Part print with two shaded views. Sizes in mm from the minimum x, y, z corner. Coordinates: 2 decimals unless noted, no trailing zeros. Order: outer loops, then holes, each group sorted by start corner. A loop starts at its lowest first (then second) coordinate and runs counter-clockwise, first axis right, second up.
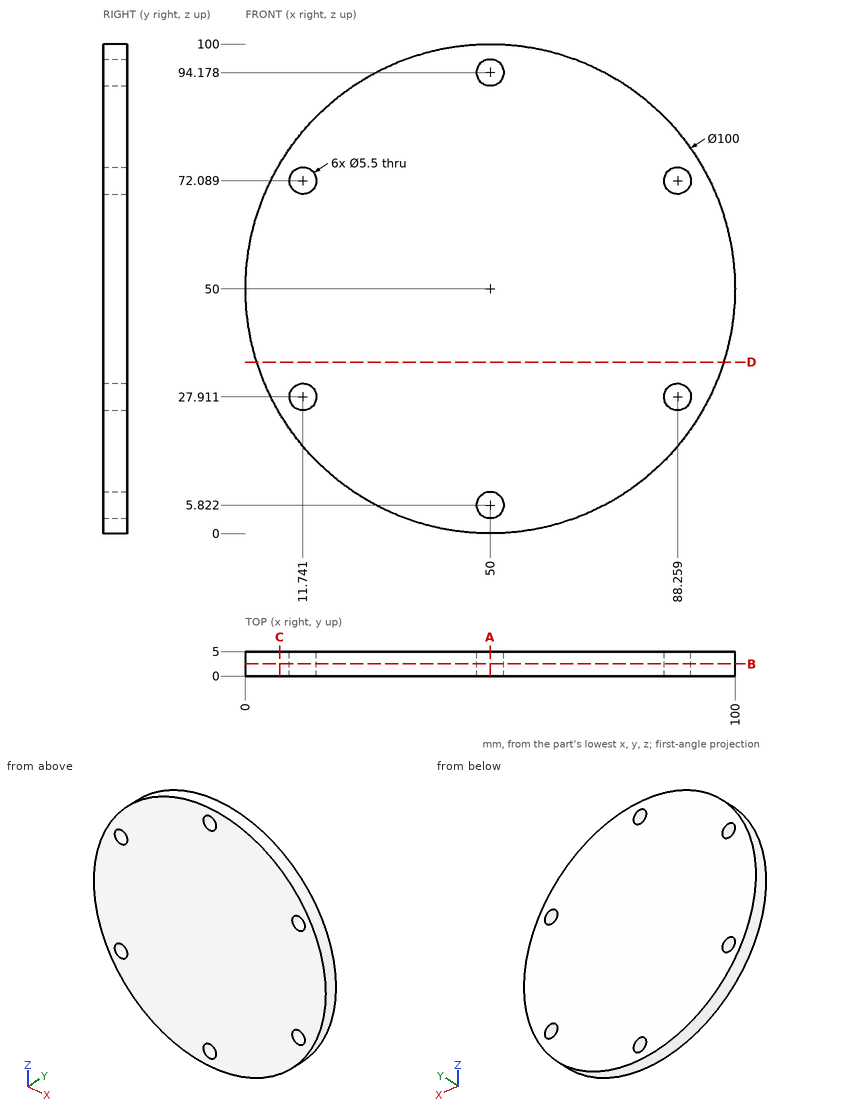
Q1. Cut at D-D on z = 35. Write the cut outline in (x, y), and give its area (3 significant figures).
Results list:
outline: (2.3, 0) - (97.7, 0) - (97.7, 5) - (2.3, 5) - close
area: 477 mm2
Q2. Cut at B-B on y = 2.5. Write the cut outline in (x, z).
Results list:
outline: circle Ø100 at (50, 50); hole circle Ø5.5 at (11.74, 27.91); hole circle Ø5.5 at (11.74, 72.09); hole circle Ø5.5 at (50, 5.82); hole circle Ø5.5 at (50, 94.18); hole circle Ø5.5 at (88.26, 27.91); hole circle Ø5.5 at (88.26, 72.09)
Q3. Cut at A-A on x = 50. Write the cut outline in (y, z).
Results list:
outline: (0, 0) - (5, 0) - (5, 3.07) - (0, 3.07) - close; (0, 8.57) - (5, 8.57) - (5, 91.43) - (0, 91.43) - close; (0, 96.93) - (5, 96.93) - (5, 100) - (0, 100) - close
Q4. Pin check, flat tips, straight feed: pin 1 Ø3.5 at (x, z) = (50, 5.82) entering from -Y; pin 2 Ø1.5 at (y, z) = (0.5, 59.5) entering from +X. Stop position of each tip, or through.
Results list:
pin 1: passes through
pin 2: stops at x = 99.23
Q5. Wall check: line 1 along Z through (x, y) = (50, 3.6); line 2 along X through (y, z) = (4.5, 27) (1 decimal); line 3 along X through (y, z) = (3, 50.5). Give the ranges that are in metal, low to high.
Results list:
line 1: z = 0 to 3.07, 8.57 to 91.43, 96.93 to 100
line 2: x = 5.6 to 9.1, 14.3 to 85.7, 90.9 to 94.4
line 3: x = 0 to 100
Q6. Cut at C-C on x = 7. Write the cut outline in (y, z) (1 decimal), and give its area (3 significant figures).
Results list:
outline: (0, 24.5) - (5, 24.5) - (5, 75.5) - (0, 75.5) - close
area: 255 mm2
